from build123d import *

# Parameters (mm, degrees)
BOSS_EXTRUDE1_DEPTH = 1003.3
CUT_EXTRUDE1_REACH  = 1006.525
SKETCH2_R           = 3.175
SKETCH3_W           = 50.8
SKETCH3_H           = 12.7
CUT_EXTRUDE2_DEPTH  = 1005.525043242


with BuildPart() as part:
    # Sketch1 → Boss-Extrude1 (new body)
    with BuildSketch(Plane.XY):
        Polygon((0, 0), (0, 38.1), (6.35, 38.1), (6.35, 6.35), (38.1, 6.35), (38.1, 0), align=None)
    extrude(amount=BOSS_EXTRUDE1_DEPTH)

    # Sketch2 → Cut-Extrude1 (cut, up to next)
    with BuildSketch(Plane(origin=(6.35, 0, 0), x_dir=(0, 0, -1), z_dir=(1, 0, 0)), mode=Mode.PRIVATE) as cut_extrude1_sk1:
        with BuildLine():
            Line((-515.9375, 38.1), (-515.9375, 25.4))
            ThreePointArc((-515.9375, 25.4), (-501.65, 11.1125), (-487.3625, 25.4))
            Line((-487.3625, 25.4), (-487.3625, 38.1))
            Line((-487.3625, 38.1), (-515.9375, 38.1))
        make_face()
    cut_extrude1_tool1 = extrude(cut_extrude1_sk1.sketch, amount=-CUT_EXTRUDE1_REACH, mode=Mode.PRIVATE) & part.part
    # Sketch2 → Cut-Extrude1 (cut, up to next)
    with BuildSketch(Plane(origin=(6.35, 0, 0), x_dir=(0, 0, -1), z_dir=(1, 0, 0)), mode=Mode.PRIVATE) as cut_extrude1_sk2:
        with Locations(Location((-527.05, 25.4, 0), (0, 0, 90))):
            Circle(SKETCH2_R)
    cut_extrude1_tool2 = extrude(cut_extrude1_sk2.sketch, amount=-CUT_EXTRUDE1_REACH, mode=Mode.PRIVATE) & part.part
    # Sketch2 → Cut-Extrude1 (cut, up to next)
    with BuildSketch(Plane(origin=(6.35, 0, 0), x_dir=(0, 0, -1), z_dir=(1, 0, 0)), mode=Mode.PRIVATE) as cut_extrude1_sk3:
        with Locations((-476.25, 25.4)):
            Circle(SKETCH2_R)
    cut_extrude1_tool3 = extrude(cut_extrude1_sk3.sketch, amount=-CUT_EXTRUDE1_REACH, mode=Mode.PRIVATE) & part.part
    add(cut_extrude1_tool1.solids().sort_by_distance((6.35, 25.926758, 501.65))[0], mode=Mode.SUBTRACT)
    add(cut_extrude1_tool2.solids().sort_by_distance((6.35, 25.4, 527.05))[0], mode=Mode.SUBTRACT)
    add(cut_extrude1_tool3.solids().sort_by_distance((6.35, 25.4, 476.25))[0], mode=Mode.SUBTRACT)

    # Sketch3 → Cut-Extrude2 (cut, through all)
    with BuildSketch(Plane(origin=(6.35, 0, 0), x_dir=(0, 0, -1), z_dir=(1, 0, 0))):
        with Locations((-25.4, 31.75)):
            Rectangle(SKETCH3_W, SKETCH3_H)
        with Locations((-977.9, 31.75)):
            Rectangle(SKETCH3_W, SKETCH3_H)
    extrude(amount=-CUT_EXTRUDE2_DEPTH, mode=Mode.SUBTRACT)


solid = part.part
Model file for the job. Use its own axes, mm. A direction names the side the tool comes from. Give positions to 0.01 mm unless a question says otherwise; leave off trailing zeros. Order: outer loops, then holes, each group sorted by start corner. A loop starts at its lowest first (then second) coordinate and runs counter-clockwise, first axis right, second up. Notation, with made-up numbers: (4.25, 66) - (40.25, 66) arc R7 ccw to (40.25, 71) - close; hole circle Ø5 at (46, 24.5). An arc over 180 degrees is marked (long way). Write item = value, one per line. Start each with the question number.
1. Which spindle directions (+Z, -Z, +X, -X, +Y, -Y) get a long thin tool onto all of the face, cutting with end or side? Do faces 1 (the flat face through (19, 0, 495)), 2 (the flat face through (6.35, 12, 495)). Say none if no direction does.
2. Probe line 1 along Z through (x, y) = (4, 25); line 2 along Z through (x, y) = (5.5, 36.5); line 3 along X through (y, z) = (16, 223). List the from-to ranges inside material, lowest first.
3. Drop flat-ended pins along their axis: P1, Ø7, axis at x = 2, z = 973, coming from the +Y side; P2, Ø5, axis at x = 4, y = 34.5, coming from the +Z side; P3, Ø9.5, axis at x = 30, z = 580, coming from the +Y side; P4, Ø5.5, axis at y = 25.4, z = 476.25, coming from the -X side. Give the stop position or say it passes through.
4. Cut at A-A, the plane z = 501.65. List the corners of the cut face in (x, y), and give its area (3 significant figures).
5. Cut at B-B, the plane x = 26.5. List the corners of the cut face in (y, z).
6. Cut at C-C, the plane z = 784. List the corners of the cut face in (x, y).
Taken from the geometry:
q1.face_1 = +Z, -Z, +X, -X, -Y
q1.face_2 = +Z, -Z, +X, +Y
q2.line_1 = 0 to 473.1, 479.4 to 487.37, 515.93 to 523.9, 530.2 to 1003.3
q2.line_2 = 50.8 to 487.36, 515.94 to 952.5
q2.line_3 = 0 to 6.35
q3.P1 = 25.4
q3.P2 = 952.5
q3.P3 = 6.35
q3.P4 = through
q4.outline = (0, 0) - (38.1, 0) - (38.1, 6.35) - (6.35, 6.35) - (6.35, 11.11) - (0, 11.11) - close
q4.area = 272 mm²
q5.outline = (0, 0) - (6.35, 0) - (6.35, 1003.3) - (0, 1003.3) - close
q6.outline = (0, 0) - (38.1, 0) - (38.1, 6.35) - (6.35, 6.35) - (6.35, 38.1) - (0, 38.1) - close
